Geometry: see drawing. Coordinates: mm, zero at the bounding-box minimum. A direction names the side the tool comes from. Give positions to 0.01 mm unless a question says otherwise; leave off trailing zeros. Order: outer loops, then holes, each group sorted by start corner. A loop starts at its lowest first (then second) coordinate and runs counter-clockwise, first axis right, second up. Notation, with made-up numbers: M 49,18 L 80,18 A17 ccw 80,47 Z; hole C 69,76.5 d3. An arc over 180 degrees is marked long. Answer as a JSON object with one key per item and string values. Group by question number.
1. Set-up query: the marked faces 1 and 2. Return all of +Z, -Z, +X, -X, +Y, -Y with unobstructed straight access to the full face (end or side cutting, diameter ignored); none if empty.
2. Pin query (flat end, axial travel): P1, Ø1, axis at y = 14, z = 16.5, coming from the +X side; P2, Ø10, axis at x = 3, z = 5, coming from the +Y side; P3, Ø4, axis at x = 9.5, y = 44.5, coming from the -Z side. Return the tip coordinate at first contact, or that it passes through.
3. Section query A-A (y = 6.5). Output: boundary loops of the cut face in (x, z), plus the area to 3 significant figures.
4. Section query B-B (y = 12). Output: boundary loops of the cut face in (x, z), plus the area to 3 significant figures.
5. Material intervals for L1, parallel to X at y = 36, z = 13; L2, parallel to Y at x = 14.5, z = 13; L3, parallel to Y at x = 16, z = 2.5, sorted ascending. Write a range as [from, to].
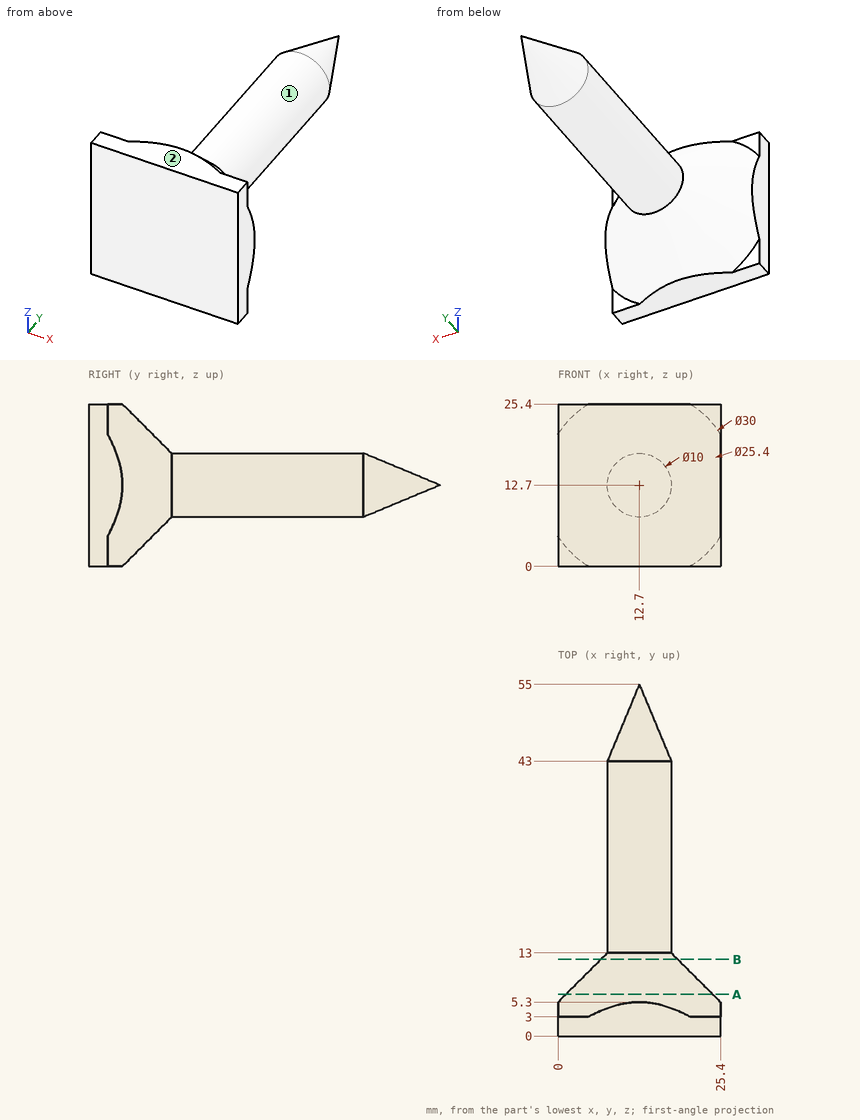
Answer sheet:
{
 "1": {"face 1": "+Y", "face 2": "+Z, +X, -X, +Y, -Y"},
 "2": {"P1": "x = 16.46", "P2": "y = 10.62", "P3": "z = 8.07"},
 "3": {"outline": "C 12.7,12.7 d23", "area": "415 mm^2"},
 "4": {"outline": "C 12.7,12.7 d12", "area": "113 mm^2"},
 "5": {"L1": "[7.71, 17.69]", "L2": "[0, 50.62]", "L3": "[0, 7.28]"}
}
